Source: CAD feature listing. Evaluate the final solid. Frame: model axes, mm. Give positions to 0.01 mm unless a question says otherwise; leave off trailing zeros. Order: outer loops, then holes, each group sorted by start corner. A loop starts at its lowest first (then second) coordinate and runs counter-clockwise, first axis right, second up.
```python
from build123d import *

# Parameters (mm, degrees)
SKETCH1_R           = 1
BOSS_EXTRUDE1_DEPTH = 2


with BuildPart() as part:
    # Sketch1 → Boss-Extrude1 (new body)
    with BuildSketch(Plane(origin=(0, 0, 0), x_dir=(1, 0, 0), z_dir=(0, 1, 0))):
        with BuildLine():
            Line((-50, -63.396226415), (-50, 54.103773585))
            ThreePointArc((-50, 54.103773585), (-49.267766953, 55.871540538), (-47.5, 56.603773585))
            Line((-47.5, 56.603773585), (-39.652542771, 56.603773585))
            ThreePointArc((-39.652542771, 56.603773585), (-38.021337196, 55.998283646), (-37.180274472, 54.475108283))
            Line((-37.180274472, 54.475108283), (-22.507731701, -43.211594583))
            ThreePointArc((-22.507731701, -43.211594583), (-22.486942565, -43.396744894), (-22.48, -43.582929282))
            Line((-22.48, -43.582929282), (-22.48, -63.396226415))
            Line((-22.48, -63.396226415), (-22.48, -78.396226415))
            Line((-22.48, -78.396226415), (-22.48, -80.896226415))
            ThreePointArc((-22.48, -80.896226415), (-23.212233047, -82.663993368), (-24.98, -83.396226415))
            Line((-24.98, -83.396226415), (-47.5, -83.396226415))
            ThreePointArc((-47.5, -83.396226415), (-49.267766953, -82.663993368), (-50, -80.896226415))
            Line((-50, -80.896226415), (-50, -78.396226415))
            Line((-50, -78.396226415), (-50, -63.396226415))
        make_face()
        with Locations((-36.24, -78.396226415)):
            Circle(SKETCH1_R, mode=Mode.SUBTRACT)
        with Locations((-45, -63.396226415)):
            Circle(SKETCH1_R, mode=Mode.SUBTRACT)
        with Locations((-27.48, -63.396226415)):
            Circle(SKETCH1_R, mode=Mode.SUBTRACT)
        with Locations((-45, -38.396226415)):
            Circle(SKETCH1_R, mode=Mode.SUBTRACT)
        with Locations((-45, 51.603773585)):
            Circle(SKETCH1_R, mode=Mode.SUBTRACT)
        with BuildLine():
            Line((-44.38816659, -42.832929282), (-31.88816659, -42.832929282))
            ThreePointArc((-31.88816659, -42.832929282), (-31.13816659, -43.582929282), (-31.88816659, -44.332929282))
            Line((-31.88816659, -44.332929282), (-44.38816659, -44.332929282))
            ThreePointArc((-44.38816659, -44.332929282), (-45.13816659, -43.582929282), (-44.38816659, -42.832929282))
        make_face(mode=Mode.SUBTRACT)
    extrude(amount=BOSS_EXTRUDE1_DEPTH)


solid = part.part
```
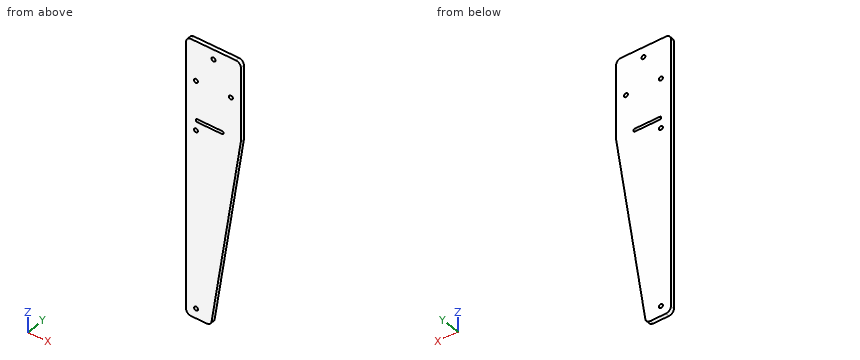
1) Pin query (flat end, axial travel): pin 1 (10 mm diameter, centred on x = -35, z = 14.5, fed in from -Y). Return the tip coordinate at first contact, or that it passes through.
Report:
pin 1: stops at y = 0
2) Section query C-C, the plane z = -36.5. Return the cut outline in (x, y).
Report:
outline: (-50, 0) - (-34.48, 0) - (-34.48, 2) - (-50, 2) - close
3) Section query B-B, the plane z = -20. Return the cut outline in (x, y), and give its area (3 significant figures).
Report:
outline: (-50, 0) - (-32, 0) - (-32, 2) - (-50, 2) - close
area: 36.0 mm2
4) Material intervals for L1, parallel to Z at x = -45, y = 1.1; L2, parallel to Z at x = -41.25, y = 0.35; L3, parallel to X at y = 0.55, z = -13, sorted ascending.
Report:
L1: z = -56.6 to -52.6, -50.6 to 37.4, 39.4 to 43.15, 44.02 to 62.4, 64.4 to 83.4
L2: z = -56.6 to 42.83, 44.33 to 83.4
L3: x = -50 to -30.95
5) Section query A-A, the plane y = 1.05. Return the cut outline in (x, z).
Report:
outline: (-50, -54.1) arc R2.5 ccw to (-47.5, -56.6) - (-39.65, -56.6) arc R2.5 ccw to (-37.18, -54.48) - (-22.51, 43.21) arc R2.5 ccw to (-22.48, 43.58) - (-22.48, 80.9) arc R2.5 ccw to (-24.98, 83.4) - (-47.5, 83.4) arc R2.5 ccw to (-50, 80.9) - close; hole circle Ø2 at (-45, -51.6); hole circle Ø2 at (-45, 38.4); hole circle Ø2 at (-45, 63.4); hole (-44.39, 42.83) - (-31.89, 42.83) arc R0.75 ccw to (-31.89, 44.33) - (-44.39, 44.33) arc R0.75 ccw to start; hole circle Ø2 at (-36.24, 78.4); hole circle Ø2 at (-27.48, 63.4)
